Autodesk Inventor part; units mm, degrees
ref_plane "YZ Plane" through (0, 0, 0) normal (1, 0, 0) x (0, 1, 0)
ref_plane "XZ Plane" through (0, 0, 0) normal (0, 1, 0) x (-1, 0, 0)
ref_plane "XY Plane" through (0, 0, 0) normal (0, 0, 1) x (1, 0, 0)
sketch "Sketch1" plane through (0, 0, 0) normal (0, 0, 1) x (1, 0, 0)
  line L0 (12.5, -19) -> (-12.5, -19)
  line L1 (-12.5, -19) -> (-12.5, 19)
  line L2 (-12.5, 19) -> (12.5, 19)
  line L3 (12.5, 19) -> (12.5, -19)
  line L4 (12.5, -19) -> (-12.5, 19) construction
  line L5 (-12.5, -19) -> (12.5, 19) construction
  circle A0 centre (0, 12.5) radius 2.1
  circle A1 centre (0, -12.5) radius 2.1
  point P0 (0, 0)
  dimension "d0" = 25
  dimension "d1" = 38
  dimension "d2" = 4.2
  dimension "d3" = 4.2
  dimension "d4" = 12.5
  dimension "d5" = 12.5
extrude "Extrusion1" add sketch "Sketch1" along normal blind 10
sketch "Sketch2" plane through (-12.5, 19, 0) normal (0, 1, 0) x (1, 0, 0)
  line L0 (0, 0) -> (0, -10)
  line L1 (0, -10) -> (-6.5, -10)
  line L2 (-6.5, -10) -> (0, 0)
  line L3 (0, -10) -> (25, -10)
  line L4 (0, 0) -> (0, -10)
  line L5 (25, -10) -> (31.5, -10)
  line L6 (25, 0) -> (25, -10)
  line L7 (31.5, -10) -> (25, 0)
  line L8 (25, 0) -> (25, -10)
  point P0 (12.5, 0)
  dimension "d8" = 6.5
  dimension "d9" = 6.5
extrude "Extrusion2" add sketch "Sketch2" against normal up to surface (38 mm away)
sketch "Sketch3" plane through (0, 0, 10) normal (0, 0, 1) x (1, 0, 0)
  line L0 (-5.4088, 0) -> (7.7062, 0)
  line L1 (0, 5.8117) -> (0, -6.6687)
  point P0 (0, 0)
  point P1 (-16, 16)
  point P2 (16, 16)
  point P3 (-16, -16)
  point P4 (16, -16)
  dimension "d12" = 16
  dimension "d13" = 16
  dimension "d16" = 32
  dimension "d19" = 32
hole "Hole1" at (-16, 16, 10) at (16, 16, 10) at (-16, -16, 10) at (16, -16, 10) direction (0, 0, -1) diameter 2.5 depth 20 tip angle 118
hole "Hole2" at (0, -12.5, 10) direction (0, 0, -1) diameter 8 depth 6 tip angle 118
hole "Hole3" at (0, 12.5, 10) direction (0, 0, -1) diameter 8 depth 6 tip angle 118
properties part number "RDtoRC2-height10mm"
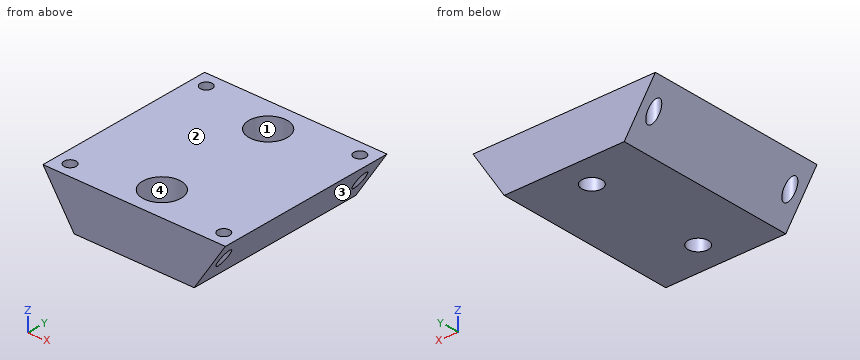
Source: CAD feature listing. Evaluate the final solid. Frame: model axes, mm. Face numbers are marked on the shaded views. Round coordinates to 2 decimals unless told otherwise and drop trailing zeros. Loops run counter-clockwise (first coordinate to the right, second up) from the corner with the lowest first, then second, coordinate; pieces in that order, holes last. Notation, with made-up numbers: M -19,43 L -10,43 A34 cw -10,78 Z; hole C -19.75,-28.5 d1. An arc over 180 degrees is marked long. Use a Markdown table: item, result. Add a question column.
1. Contact query for flat-ended pins moving along their axis: pin 1 (3 mm diameter, centred on x = -16, y = 16, fed in from -Z); pin 2 (1.5 mm diameter, centred on x = -16, y = -16, fed in from -Z); pin 3 (6 mm diameter, centred on y = 9.5, z = 2.5, fed in from -X) (3 decimals); pin 4 (2 mm diameter, centred on y = -4.5, z = 6.5, fed in from -X) (3 decimals). Output: stop coordinate, or through.
2. Cut plane C-C, the plane z = 8.75. Output: boundary loops of the cut face in (x, y).
3. Ray query, line 1 along Y through (x, z) = (0, 6.25); line 2 along Y through (x, z) = (0, 0.65); line 3 along X through (y, z) = (-16, 7.75). Return the intervals inside material, ascending. Write a range as [from, to].
4. Cut plane B-B, the plane x = 16. Output: boundary loops of the cut face in (y, z), and give its area (3 significant figures).
5. Cut plane A-A, the plane y = 12.5. Output: boundary loops of the cut face in (x, z), and give its area (3 significant figures).
6. Pull-direction query (X, two-part tool) for the marked faces 1, 2, 3 and 4; classes: +X half, -X half, draft (parallel to the pull), parting line (faces both ways), or undercut.
7. Cut plane D-D, the plane z = 4.5. Output: boundary loops of the cut face in (x, y) (3 decimals).
Solution:
| question | item | result |
|---|---|---|
| 1 | pin 1 | stops at z = 3.08 |
| 1 | pin 2 | passes through |
| 1 | pin 3 | stops at x = -16.075 |
| 1 | pin 4 | stops at x = -17.375 |
| 2 | outline | M -18.19,-19 L 18.19,-19 L 18.19,19 L -18.19,19 Z; hole C -16,-16 d2.5; hole C -16,16 d2.5; hole C 0,-12.5 d8; hole C 0,12.5 d8; hole C 16,-16 d2.5; hole C 16,16 d2.5 |
| 3 | line 1 | y = [-19, -16.5], [-8.5, 8.5], [16.5, 19] |
| 3 | line 2 | y = [-19, -14.6], [-10.4, 10.4], [14.6, 19] |
| 3 | line 3 | x = [-17.54, -17.25], [-14.75, -1.94], [1.94, 14.75], [17.25, 17.54] |
| 4 | outline | M -19,5.38 L -17.25,5.38 L -17.25,10 L -19,10 Z; M -14.75,5.38 L 14.75,5.38 L 14.75,10 L -14.75,10 Z; M 17.25,5.38 L 19,5.38 L 19,10 L 17.25,10 Z |
| 4 | area | 152 mm2 |
| 5 | outline | M -19,10 L -12.5,0 L -2.1,0 L -2.1,2.86 L -4,4 L -4,10 Z; M 2.1,0 L 12.5,0 L 19,10 L 4,10 L 4,4 L 2.1,2.86 Z |
| 5 | area | 248 mm2 |
| 6 | face 1 | undercut |
| 6 | face 2 | draft |
| 6 | face 3 | +X half |
| 6 | face 4 | undercut |
| 7 | outline | M -15.425,-19 L 15.425,-19 L 15.425,-17.11 A1.25 cw 15.425,-14.89 L 15.425,14.89 A1.25 cw 15.425,17.11 L 15.425,19 L -15.425,19 L -15.425,17.11 A1.25 cw -15.425,14.89 L -15.425,-14.89 A1.25 cw -15.425,-17.11 Z; hole C 0,-12.5 d8; hole C 0,12.5 d8 |
